from build123d import *

# Parameters (mm, degrees)
SKETCH_1_W          = 40
SKETCH_1_H          = 21
EXTRUDE_1_DEPTH     = 1.5
SKETCH_2_R          = 0.7
SKETCH_2_R_2        = 0.5
SKETCH_2_R_3        = 0.35
SKETCH_2_R_4        = 1.6
CUT_EXTRUDE_1_DEPTH = 2.5


with BuildPart() as part:
    # Эскиз1 → Бобышка-Вытянуть1 (new body)
    with BuildSketch(Plane(origin=(0, 0, 0), x_dir=(1, 0, 0), z_dir=(0, 1, 0))):
        with Locations((20, 10.5)):
            Rectangle(SKETCH_1_W, SKETCH_1_H)
    extrude(amount=EXTRUDE_1_DEPTH)

    # Эскиз2 → Вырез-Вытянуть1 (cut, through all)
    with BuildSketch(Plane(origin=(0, 1.5, 0), x_dir=(1, 0, 0), z_dir=(0, 1, 0))):
        with Locations((29.5, 3.5)):
            Circle(SKETCH_2_R)
        with Locations((27, 3.5)):
            Circle(SKETCH_2_R_2)
        with Locations((13, 3.5)):
            Circle(SKETCH_2_R)
        with Locations((10.5, 3.5)):
            Circle(SKETCH_2_R_2)
        with Locations((27, 6)):
            Circle(SKETCH_2_R_3)
        with Locations((29.5, 6)):
            Circle(SKETCH_2_R_3)
        with Locations((29.5, 1)):
            Circle(SKETCH_2_R_3)
        with Locations((27, 1)):
            Circle(SKETCH_2_R_3)
        with Locations((13, 6)):
            Circle(SKETCH_2_R_3)
        with Locations((10.5, 6)):
            Circle(SKETCH_2_R_3)
        with Locations((10.5, 1)):
            Circle(SKETCH_2_R_3)
        with Locations((13, 1)):
            Circle(SKETCH_2_R_3)
        with Locations((3, 10)):
            Circle(SKETCH_2_R_4)
        with Locations((37, 10)):
            Circle(SKETCH_2_R_4)
        with Locations((3, 15)):
            Circle(SKETCH_2_R_4)
        with Locations((37, 15)):
            Circle(SKETCH_2_R_4)
    extrude(amount=-CUT_EXTRUDE_1_DEPTH, mode=Mode.SUBTRACT)


solid = part.part
Could you check a few things on this model? Use its own coordinates, in mm. Give positions to 0.01 mm unless a question says otherwise; leave off trailing zeros. Write each loop counter-clockwise with the first axis right and the second up, starting at its lowest first coordinate (ties: lowest second). Pieces come first, ordered by that corner, then holes. Notation, with made-up numbers: (55.5, -39.5) -> (92.5, -39.5) arc R17 cw to (92.5, -12.5) -> close; hole circle Ø7 at (61, 17). An arc over 180 degrees is marked (long way). Answer as a JSON object with one key per item and string values.
Q1. Please list where these lines run through material, in increasing order: L1, parallel to X at y = 1.05, z = -10; L2, parallel to Z at x = 3, y = 0.65; L3, parallel to X at y = 0.8, z = -6.
Taken from the geometry:
{"L1": "x = 0 to 1.4, 4.6 to 35.4, 38.6 to 40", "L2": "z = -21 to -16.6, -13.4 to -11.6, -8.4 to 0", "L3": "x = 0 to 10.15, 10.85 to 12.65, 13.35 to 26.65, 27.35 to 29.15, 29.85 to 40"}
Q2. Suppose I cut it at A-A on z = -3.5. Write out the boundary of the cut face in (x, y).
Taken from the geometry:
{"outline": "(0, 0) -> (10, 0) -> (10, 1.5) -> (0, 1.5) -> close; (11, 0) -> (12.3, 0) -> (12.3, 1.5) -> (11, 1.5) -> close; (13.7, 0) -> (26.5, 0) -> (26.5, 1.5) -> (13.7, 1.5) -> close; (27.5, 0) -> (28.8, 0) -> (28.8, 1.5) -> (27.5, 1.5) -> close; (30.2, 0) -> (40, 0) -> (40, 1.5) -> (30.2, 1.5) -> close"}
Q3. Suppose I cut it at B-B on x = 3. Write out the boundary of the cut face in (y, z).
Taken from the geometry:
{"outline": "(0, -21) -> (1.5, -21) -> (1.5, -16.6) -> (0, -16.6) -> close; (0, -13.4) -> (1.5, -13.4) -> (1.5, -11.6) -> (0, -11.6) -> close; (0, -8.4) -> (1.5, -8.4) -> (1.5, 0) -> (0, 0) -> close"}
Q4. Suppose I cut it at D-D on y = 1.05. Count the separate pieces of the cut face and the enclosed holes in it, then the cut area to 3 significant figures.
Taken from the geometry:
{"separate pieces": "1", "enclosed holes": "16", "area": "800 mm²"}
Q5. Suppose I cut it at C-C on z = -10. Write out the boundary of the cut face in (x, y), then the cut area to 3 significant figures.
Taken from the geometry:
{"outline": "(0, 0) -> (1.4, 0) -> (1.4, 1.5) -> (0, 1.5) -> close; (4.6, 0) -> (35.4, 0) -> (35.4, 1.5) -> (4.6, 1.5) -> close; (38.6, 0) -> (40, 0) -> (40, 1.5) -> (38.6, 1.5) -> close", "area": "50.4 mm²"}
Q6. We'd pull the mould along Z, two halves only. Please class faces 1 (the cylindrical face through (2.65, 0.76, -8.44)), 2 (the flat face through (20, 0, -11)), 3 (the flat face through (20, 1, 0)): released by +Z, released by -Z, zero draft, split by the parting line, or undercut.
Taken from the geometry:
{"face 1": "undercut", "face 2": "zero draft", "face 3": "released by +Z"}
